Build history of the part. All positions in model axes, mm. A direction names the side the tool comes from. Give positions to 0.01 mm unless a question says otherwise; leave off trailing zeros. Write each loop counter-clockwise with the first axis right and the second up, starting at its lowest first coordinate (ties: lowest second). Pieces come first, ordered by that corner, then holes. Notation, with made-up numbers: (72.25, 66.5) -> (98.25, 66.5) arc R24 ccw to (98.25, 95.5) -> close; hole circle Ø7 at (19.5, 14). An arc over 180 degrees is marked (long way). One line per question, with ' | ' between items. Start each with the question number.
(1) Pin check, flat tips, straight feed: P1, Ø1.5, axis at x = 24.5, z = 2, coming from the +Y side; P2, Ø2.5, axis at x = 29, y = 4.5, coming from the +Z side. Stop position of each tip, or through.
(2) Band-saw the part on D-D, the plane x = 13. Give the cut face in (y, z).
(3) Band-saw the part on A-A, the plane x = 19. Give the cut face in (y, z), and give its area (3 significant figures).
(4) Band-saw the part on B-B, the plane y = 3.5. Give the cut face in (x, z).
(5) Pull direction Y, two halves, no side cores. Call faces 1 (the flat face through (24.74, 7.74, 1)), 2 (the flat face through (8, 5, 2.032)), 3 (the cylindrical face through (0, 4.4, 1)), 4 (the cylindrical face through (17.908, 1.417, 2.318)): released by +Y, released by -Y, zero draft, split by the parting line, or undercut.
(6) Drill centre lines: probe 1 along X at (y, z) = (4.25, 2.55); probe 2 along Z at (x, y) = (24.5, 6.5); probe 3 along Y at (x, z) = (18.5, 1.25). Where is each one in solid material? Low to high. Write a range as from..to.
(7) Tool access for faces 5 (the flat face through (18.9, 1.5, 4.572)), 6 (the cylindrical face through (17, 0, 3)): list every direction of +Z, -Z, +X, -X, +Y, -Y with a clear straight run to the whole face (end or side of a thin tool).
Solid Edge part; units mm, degrees
sketch "Sketch1" plane through (0, 0, 0) normal (0, 0, 1) x (1, 0, 0)
  line L0 (16.2788, 8.8383) -> (1.8566, 6.6201)
  line L1 (1.8533, 2.2927) -> (16.2721, 0.0527)
  line L2 (17.6335, 0.0522) -> (32.0541, 2.2813)
  line L3 (17.6335, 8.8378) -> (32.0541, 6.6087)
  arc A0 (16.2788, 8.8383) -> (17.6335, 8.8378) centre (16.9545, 4.445) cw
  arc A1 (1.8566, 6.6201) -> (1.8533, 2.2927) centre (2.1894, 4.4561) ccw
  arc A2 (16.2721, 0.0527) -> (17.6335, 0.0522) centre (16.9545, 4.445) ccw
  arc A3 (32.0541, 2.2813) -> (32.0541, 6.6087) centre (31.7196, 4.445) ccw
  dimension "D1" = 33.909
extrude "Protrusion1" add sketch "Sketch1" along normal blind 2.032
sketch "Sketch2" plane through (16.9545, 4.445, 2.032) normal (0, 0, 1) x (0.9884, 0.152, 0)
  circle A0 centre (0, 0) radius 4.445
extrude "ExtrudedProtrusion_2" add sketch "Sketch2" along normal blind 2.54
hole "Hole_1" at (16.9545, 4.445, 4.572) direction (0, 0, -1) diameter 6.35 end up to next
properties part number "HARDWARE"
Results:
1) P1: stops at y = 7.89 | P2: stops at z = 2.03
2) outline: (0.56, 0) -> (8.33, 0) -> (8.33, 2.03) -> (6.47, 2.03) -> (6.47, 4.57) -> (2.42, 4.57) -> (2.42, 2.03) -> (0.56, 2.03) -> close
3) outline: (0.26, 0) -> (2.02, 0) -> (2.02, 4.57) -> (0.5, 4.57) -> (0.5, 2.03) -> (0.26, 2.03) -> close; (6.87, 0) -> (8.63, 0) -> (8.63, 2.03) -> (8.39, 2.03) -> (8.39, 4.57) -> (6.87, 4.57) -> close | area: 14.8 mm²
4) outline: (0.22, 0) -> (13.92, 0) -> (13.92, 4.57) -> (12.61, 4.57) -> (12.61, 2.03) -> (0.22, 2.03) -> close; (19.99, 0) -> (33.69, 0) -> (33.69, 2.03) -> (21.3, 2.03) -> (21.3, 4.57) -> (19.99, 4.57) -> close
5) face 1: released by +Y | face 2: zero draft | face 3: split by the parting line | face 4: undercut
6) probe 1: x = 12.51..13.79, 20.12..21.4 | probe 2: z = 0..2.03 | probe 3: y = 0.19..1.67, 7.22..8.7
7) face 5: +Z, +X, -X, +Y, -Y | face 6: +Z
